Geometry: final body of the model. Coordinates: model frame, mm. A direction names the side the tool comes from. Coordinates: 2 decimals unless noted, no trailing zeros. Order: outer loops, then holes, each group sorted by start corner. A loop starts at its lowest first (then second) coordinate and runs counter-clockwise, first axis right, second up. Notation, with made-up numbers: M -1,-27 L 55,-27 A26 cw 55,-10 Z; hole C -28.75,18 d7. An arc over 180 degrees is marked long. Write item = value, one per line.
Autodesk Inventor part; units mm, degrees
ref_plane "YZ Plane" through (0, 0, 0) normal (1, 0, 0) x (0, 1, 0)
ref_plane "XZ Plane" through (0, 0, 0) normal (0, 1, 0) x (-1, 0, 0)
ref_plane "XY Plane" through (0, 0, 0) normal (0, 0, 1) x (1, 0, 0)
sketch "Szkic1" plane through (0, 0, 0) normal (0, 0, 1) x (1, 0, 0)
  line L0 (-10.2233, 17.3341) -> (-10.2233, -75.2659)
  line L1 (-10.2233, -75.2659) -> (31.7767, -75.2659)
  line L2 (-10.2233, 17.3341) -> (31.7767, 17.3341)
  line L3 (31.7767, 17.3341) -> (31.7767, -7.9659)
  line L4 (31.7767, -75.2659) -> (31.7767, -49.9659)
  line L5 (31.7767, -49.9659) -> (77.7767, -49.9659)
  line L6 (77.7767, -49.9659) -> (77.7767, -7.9659)
  line L7 (77.7767, -7.9659) -> (31.7767, -7.9659)
  point P0 (0, 0)
  point P1 (41.2767, -13.4659)
  point P2 (72.2767, -13.4659)
  point P3 (41.2767, -44.4659)
  point P4 (72.2767, -44.4659)
  point P5 (56.7767, -28.9659)
  point P6 (-4.4733, 12.3341)
  point P7 (26.0267, 12.3341)
  point P8 (-4.4733, -13.6659)
  point P9 (26.0267, -13.6659)
  point P10 (-4.4733, -44.2659)
  point P11 (26.0267, -44.2659)
  point P12 (-4.4733, -70.2659)
  point P13 (26.0267, -70.2659)
  dimension "d0" = 92.6
  dimension "d1" = 42
  dimension "d2" = 42
  dimension "d3" = 46
  dimension "d4" = 25.3
  dimension "d11" = 15.5
  dimension "d12" = 15.5
  dimension "d14" = 15.5
  dimension "d15" = 15.5
  dimension "d16" = 15.5
  dimension "d17" = 15.5
  dimension "d18" = 15.5
  dimension "d19" = 15.5
  dimension "d20" = 21
  dimension "d21" = 21
  dimension "d39" = 5
  dimension "d40" = 5
  dimension "d41" = 5
  dimension "d42" = 5
  dimension "d43" = 5.75
  dimension "d44" = 5.75
  dimension "d45" = 42
  dimension "d46" = 5.75
  dimension "d47" = 5.75
  dimension "d48" = 5.75
  dimension "d49" = 5.75
  dimension "d50" = 25.3
  dimension "d51" = 5.75
  dimension "d52" = 5.75
  dimension "d60" = 26
  dimension "d61" = 26
  dimension "d62" = 26
  dimension "d63" = 26
extrude "Wyciągnięcie proste1" add sketch "Szkic1" along normal blind 4
hole "Otwór1" at (41.2767, -13.4659, 0) at (72.2767, -13.4659, 0) at (41.2767, -44.4659, 0) at (72.2767, -44.4659, 0) direction (0, 0, 1) diameter 3 end through all
hole "Otwór2" at (56.7767, -28.9659, 0) direction (0, 0, 1) diameter 22.5 end through all
chamfer "Faza1" distance 2 angle 45 2 edges at (77.7767, -7.9659, 2) (77.7767, -49.9659, 2)
hole "Otwór3" at (-4.4733, 12.3341, 0) at (26.0267, 12.3341, 0) at (-4.4733, -13.6659, 0) at (26.0267, -13.6659, 0) at (-4.4733, -44.2659, 0) at (26.0267, -44.2659, 0) at (-4.4733, -70.2659, 0) at (26.0267, -70.2659, 0) direction (0, 0, 1) diameter 5 end through all
fillet "Zaokrąglenie1" radius 1 4 edges at (31.7767, 17.3341, 2) (-10.2233, 17.3341, 2) (31.7767, -75.2659, 2) (-10.2233, -75.2659, 2)
equation "\"d4\" = -0.5 * d2 + 0.5 * d0"
equation "\"d45\" = d1"
properties part number "LC_ALU_4mm_X_End_Motor_Side"
1) Section C-C, the plane z = 3.25. Give the number of separate pieces and of enclosed holes in the cut face, and give its area (3 significant figures).
Numbers:
separate_pieces = 1
enclosed_holes = 13
area = 5,230 mm²
2) Section A-A, the plane y = 11.5. Return loops of the section in (x, z).
Numbers:
outline = M -10.22,0 L -6.83,0 L -6.83,4 L -10.22,4 Z; M -2.12,0 L 23.67,0 L 23.67,4 L -2.12,4 Z; M 28.38,0 L 31.78,0 L 31.78,4 L 28.38,4 Z
3) Pin query (flat end, axial travel): pin 1 (1.2 mm diameter, centred on x = 63, z = 2, fed in from +Y); pin 2 (2 mm diameter, centred on x = 48, z = 2, fed in from -Y). Return the tip coordinate at first contact, or that it passes through.
Numbers:
pin_1 = -7.97
pin_2 = -49.97
4) Set-up query: faces 5 (the face through (31.777, 4, 2)), 6 (the face through (31.777, -62, 2)), 7 (the face through (23.548, -70.591, 2.028)). Return all of +Z, -Z, +X, -X, +Y, -Y with unobstructed straight access to the full face (end or side cutting, diameter ignored); none if empty.
Numbers:
face_5 = +Z, -Z, +X, +Y
face_6 = +Z, -Z, +X, -Y
face_7 = +Z, -Z
5) Section D-D, the plane y = -13. Return loops of the section in (x, z).
Numbers:
outline = M -10.22,0 L -6.88,0 L -6.88,4 L -10.22,4 Z; M -2.06,0 L 23.62,0 L 23.62,4 L -2.06,4 Z; M 28.44,0 L 39.85,0 L 39.85,4 L 28.44,4 Z; M 42.7,0 L 70.85,0 L 70.85,4 L 42.7,4 Z; M 73.7,0 L 77.78,0 L 77.78,4 L 73.7,4 Z
6) Line query: L1, parallel to X at y = 12.5, z = 2.65; L2, parallel to Y at x = 25, z = 3.35; L3, parallel to Y at x = 27, z = 2.5. Output: solid intervals per line, ascending.
Numbers:
L1 = -10.22 to -6.97, -1.98 to 23.53, 28.52 to 31.78
L2 = -75.27 to -72.55, -67.99 to -46.55, -41.99 to -15.95, -11.39 to 10.05, 14.61 to 17.33
L3 = -75.27 to -72.57, -67.96 to -46.57, -41.96 to -15.97, -11.36 to 10.03, 14.64 to 17.33
7) Section B-B, the plane y = -23. Return loops of the section in (x, z), and give its area (3 significant figures).
Numbers:
outline = M -10.22,0 L 47.24,0 L 47.24,4 L -10.22,4 Z; M 66.31,0 L 77.78,0 L 77.78,4 L 66.31,4 Z
area = 276 mm²
8) Mould query, pull axis X, two halves, no side actions, for faces 1 (the face through (40.01, -43.66, 2.03)), 2 (the face through (-5.22, 14.72, 2.03)), 3 (the face through (10, 17.334, 2)), 4 (the face through (-10.223, -28, 2)). Classes: pulls with the +X half, pulls with the -X half, needs draft (parallel to the pull), parting line crosses it, or undercut.
Numbers:
face_1 = undercut
face_2 = undercut
face_3 = needs draft
face_4 = pulls with the -X half
